Read the model definition and answer for the solid it produces. Units are mm, in the model's axes. A direction names the side the tool comes from. Coordinates: 2 decimals unless noted, no trailing zeros. Order: outer loops, then holes, each group sorted by start corner. A loop starts at its lowest first (then second) coordinate and runs counter-clockwise, first axis right, second up. Notation, with made-up numbers: M 66,1 L 84,1 A17 ccw 84,5 Z; hole C 31.5,83 d5. An arc over 180 degrees is marked long. Write each question's results on one line, items separated by ' | '.
```python
from build123d import *

# Parameters (mm, degrees)
SKETCH_1_R      = 15
EXTRUDE_1_DEPTH = 20
SKETCH_2_W      = 5
SKETCH_2_H      = 15


with BuildPart() as part:
    # 草图1 → 凸台-拉伸1 (new body)
    with BuildSketch(Plane(origin=(0, 0, 0), x_dir=(1, 0, 0), z_dir=(0, 1, 0))):
        Circle(SKETCH_1_R)
        with BuildLine():
            Line((-1, -1.118033989), (-1, 1.118033989))
            ThreePointArc((-1, 1.118033989), (1.5, 0), (-1, -1.118033989))
        make_face(mode=Mode.SUBTRACT)
    extrude(amount=EXTRUDE_1_DEPTH)

    # 草图2 → 切除-旋转1 (revolve, cut)
    with BuildSketch(Plane.XY):
        with Locations((12.5, 9.892021361)):
            Rectangle(SKETCH_2_W, SKETCH_2_H)
    revolve(axis=Axis((0, 0, 0), (0, 1, 0)), mode=Mode.SUBTRACT)


solid = part.part
```
(1) Given pin 1 (4 mm diameter, centred on y = 15.5, z = 2.5, fed in from +X); pin 2 (8 mm diameter, centred on y = 13, z = 3.5, fed in from -X); pin 3 (8 mm diameter, centred on y = 9.5, z = -7.5, fed in from -X), each flat-ended and moving along its own axis, determine where each tip first touches the part or whether it passes through.
Conclusion:
pin 1: x = 14.89 | pin 2: x = -10 | pin 3: x = -9.37
(2) The mould has two halves that part along Z. Classify faces 1 (the flat face through (-3, 2.392, 10)), 2 (the cylindrical face through (-2.17, 10, 9.76)), 3 (the flat face through (-1, 10, 0)): pulls with the +Z half, pulls with the -Z half, needs draft (parallel to the pull), parting line crosses it, or undercut.
Conclusion:
face 1: needs draft | face 2: parting line crosses it | face 3: undercut
(3) The part is cut by section A-A, the plane x = 0. Write down the section's boundary in (y, z), then the cut area to 3 significant figures.
Conclusion:
outline: M 0,-15 L 2.39,-15 L 2.39,-10 L 17.39,-10 L 17.39,-15 L 20,-15 L 20,-1.5 L 0,-1.5 Z; M 0,1.5 L 20,1.5 L 20,15 L 17.39,15 L 17.39,10 L 2.39,10 L 2.39,15 L 0,15 Z | area: 390 mm²
(4) The part is cut by section D-D, the plane x = 10.5. Write down the section's boundary in (y, z), then the cut area to 3 significant figures.
Conclusion:
outline: M 0,-10.71 L 2.39,-10.71 L 2.39,10.71 L 0,10.71 Z; M 17.39,-10.71 L 20,-10.71 L 20,10.71 L 17.39,10.71 Z | area: 107 mm²
(5) Straight lines are drawn through the part: line 1 (X direction, y = 4.25, z = 0); line 2 (Y direction, x = -8.75, z = 9.5); line 3 (Z direction, x = 0, y = 6.5). For each, find the intervals that lie inside material, in ascending order.
Conclusion:
line 1: -10 to -1, 1.5 to 10 | line 2: 0 to 2.39, 17.39 to 20 | line 3: -10 to -1.5, 1.5 to 10
(6) The part is cut by section C-C, the plane y = 8. Write down the section's boundary in (x, z), then the cut area to 3 significant figures.
Conclusion:
outline: C 0,0 d20; hole M -1,-1.12 A1.5 ccw long -1,1.12 Z | area: 308 mm²
(7) For faces 4 (the flat face through (-3, 17.392, 10)), 5 (the flat face through (3, 20, 0)), determine the directions among +Z, -Z, +X, -X, +Y, -Y from which every point of the face is accessible in a straight line to the end or side of a thin tool.
Conclusion:
face 4: none | face 5: +Z, -Z, +X, -X, +Y
(8) The part is cut by section B-B, the plane z = 0. Write down the section's boundary in (x, y), then the cut area to 3 significant figures.
Conclusion:
outline: M -15,0 L -1,0 L -1,20 L -15,20 L -15,17.39 L -10,17.39 L -10,2.39 L -15,2.39 Z; M 1.5,0 L 15,0 L 15,2.39 L 10,2.39 L 10,17.39 L 15,17.39 L 15,20 L 1.5,20 Z | area: 400 mm²
